```python
from build123d import *

# Parameters (mm, degrees)
SKETCH1_W               = 40
SKETCH1_H               = 9
BOSS_EXTRUDE1_DEPTH     = 8.28
CUT_EXTRUDE1_DEPTH      = 5
CUT_EXTRUDE1_DEPTH_BACK = 10
SKETCH2_R               = 1
SKETCH3_R               = 1.75
CUT_EXTRUDE6_DEPTH      = 3.8
SKETCH4_W               = 3.5
SKETCH4_H               = 0.5
CUT_EXTRUDE7_DEPTH      = 2.5


with BuildPart() as part:
    # Sketch1 → Boss-Extrude1 (new body)
    with BuildSketch(Plane(origin=(0, 0, 0), x_dir=(1, 0, 0), z_dir=(0, 1, 0))):
        with Locations((20, 4.5)):
            Rectangle(SKETCH1_W, SKETCH1_H)
    extrude(amount=BOSS_EXTRUDE1_DEPTH)

    # Sketch2 → Cut-Extrude1 (cut, two sides: drawn at the far end of the back side and taken through both)
    with BuildSketch(Plane(origin=(0, 8.28, 0), x_dir=(1, 0, 0), z_dir=(0, 1, 0)).offset(-CUT_EXTRUDE1_DEPTH_BACK)):
        with Locations(Location((8, 4, 0), (0, 0, 90))):
            Circle(SKETCH2_R)
        with Locations(Location((32, 4, 0), (0, 0, 90))):
            Circle(SKETCH2_R)
    extrude(amount=CUT_EXTRUDE1_DEPTH + CUT_EXTRUDE1_DEPTH_BACK, mode=Mode.SUBTRACT)

    # Sketch3 → Cut-Extrude6 (cut)
    with BuildSketch(Plane(origin=(0, 0, -9), x_dir=(-1, 0, 0), z_dir=(0, 0, -1))):
        with Locations((-32, 4.78)):
            Circle(SKETCH3_R)
        with Locations((-8, 4.78)):
            Circle(SKETCH3_R)
    extrude(amount=-CUT_EXTRUDE6_DEPTH, mode=Mode.SUBTRACT)

    # Sketch4 → Cut-Extrude7 (cut)
    with BuildSketch(Plane(origin=(0, 0, -5.2), x_dir=(-1, 0, 0), z_dir=(0, 0, -1))):
        Polygon((-30.25, 5.03), (-33.25, 5.03), (-34.25, 4.53), (-30.25, 4.53), align=None)
        with Locations((-8, 4.78)):
            Rectangle(SKETCH4_W, SKETCH4_H)
    extrude(amount=-CUT_EXTRUDE7_DEPTH, mode=Mode.SUBTRACT)


solid = part.part
```
Check sheet for the modelled part. Datum: model origin and axes. Units: mm. A direction names the side the tool comes from. Coordinates: 2 decimals unless noted, no trailing zeros. Order: outer loops, then holes, each group sorted by start corner. A loop starts at its lowest first (then second) coordinate and runs counter-clockwise, first axis right, second up. Notation, with made-up numbers: M 61.25,3 L 88.25,3 A24 cw 88.25,26 Z; hole C 75.5,77 d3. An arc over 180 degrees is marked long. One line per question, with ' | ' between items. Start each with the question number.
Item 1: Access from +Z, -Z, +X, -X, +Y, -Y to the whole of each face (thin tool, end or side, straight path). Record for faces 4 (the flat face through (8, 4, -5.2)), 5 (the cylindrical face through (31, 7, -4)), 6 (the flat face through (33.2, 4.53, -4)).
Item 2: Sectioned sample at B-B on x = 32. Record the cut outline in (y, z), and give its area (3 significant figures).
Item 3: Gauge pin test, flat end, axial feed: P1, Ø1.2, axis at x = 8, y = 4, coming from the -Z side. Record the tip position at first contact, or that the pin passes through.
Item 4: Sectioned sample at D-D on z = -8. Record the cut outline in (x, y), and give its area (3 significant figures).
Item 5: Sectioned sample at A-A on z = -4. Record the cut outline in (x, y).
Item 6: Material ranges on line 1 (X direction, y = 0.9, z = -4); line 2 (Z direction, x = 32, y = 3.4); line 3 (Y direction, x = 32, z = -6.7), recorded low to high.
Item 7: Mould release check, pull along Z, two halves, no side actions. Record for faces 1 (the cylindrical face through (31, 2, -4)), 2 (the flat face through (20, 4, 0)), 3 (the flat face through (32, 6, -5.2)): pulls with the +Z half, pulls with the -Z half, needs draft (parallel to the pull), parting line crosses it, or undercut.
Item 8: Sectioned sample at C-C on y = 1. Record the cut outline in (x, z), and give its area (3 significant figures).
Answer below:
1) face 4: -Z | face 5: +Y, -Y | face 6: none
2) outline: M 0,-9 L 3.03,-9 L 3.03,-5.2 L 4.53,-5.2 L 4.53,-5 L 0,-5 Z; M 0,-3 L 4.53,-3 L 4.53,-2.7 L 5.03,-2.7 L 5.03,-3 L 8.28,-3 L 8.28,0 L 0,0 Z; M 5.03,-5.2 L 6.53,-5.2 L 6.53,-9 L 8.28,-9 L 8.28,-5 L 5.03,-5 Z | area: 44.4 mm^2
3) P1: stops at z = -5.2
4) outline: M 0,0 L 40,0 L 40,8.28 L 0,8.28 Z; hole C 8,4.78 d3.5; hole C 32,4.78 d3.5 | area: 312 mm^2
5) outline: M 0,0 L 7,0 L 7,4.53 L 6.25,4.53 L 6.25,5.03 L 7,5.03 L 7,8.28 L 0,8.28 Z; M 9,0 L 31,0 L 31,4.53 L 30.25,4.53 L 30.25,5.03 L 31,5.03 L 31,8.28 L 9,8.28 L 9,5.03 L 9.75,5.03 L 9.75,4.53 L 9,4.53 Z; M 33,0 L 40,0 L 40,8.28 L 33,8.28 L 33,5.03 L 33.25,5.03 L 34.25,4.53 L 33,4.53 Z
6) line 1: x = 0 to 7, 9 to 31, 33 to 40 | line 2: z = -5.2 to -5, -3 to 0 | line 3: y = 0 to 3.03, 6.53 to 8.28
7) face 1: undercut | face 2: pulls with the +Z half | face 3: pulls with the -Z half
8) outline: M 0,-9 L 40,-9 L 40,0 L 0,0 Z; hole C 8,-4 d2; hole C 32,-4 d2 | area: 354 mm^2
